Check sheet for the modelled part. Datum: model origin and axes. Units: mm. Face numbers are marked on the shaded views. A direction names the side the tool comes from. Round coordinates to 2 decimals unless told otherwise and drop trailing zeros. Order: outer loops, then holes, each group sorted by start corner. A loop starts at its lowest first (then second) coordinate and runs counter-clockwise, first axis right, second up. Notation, with made-up numbers: (-40, 84.5) -> (19, 84.5) arc R25 cw to (19, 100.5) -> close; hole circle Ø8 at (63, 84.5). An arc over 180 degrees is marked (long way). Answer in a Markdown table with one row per item.
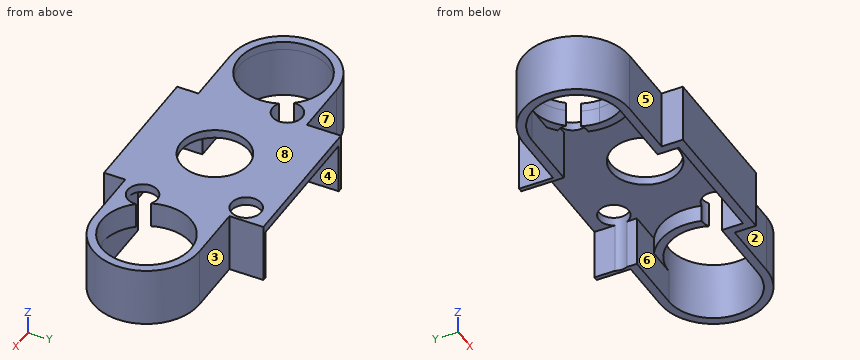
from build123d import *

# Parameters (mm, degrees)
FRONT_PLATE_DEPTH                   = 2
SHELL_DEPTH                         = 12
SHELL_HOLLOW_DEPTH                  = 12
SK_IRRINGS_R                        = 12.5
SK_IRRINGS_R_2                      = 10.5
IR_LED_RINGS_DEPTH                  = 4
LENS_LDR_AND_IR_OPENINGS_DEPTH      = 53.792538299
LENS_LDR_AND_IR_OPENINGS_DEPTH_BACK = 53.792538299
SK_FRONTOPENINGS_R                  = 8
SK_FRONTOPENINGS_R_2                = 3.5
SK_FRONTOPENINGS_R_3                = 10.5
IR_BOARD_NOTCHES_DEPTH              = 53.792538299
IR_BOARD_NOTCHES_DEPTH_BACK         = 53.792538299
SK_IRNOTCHES_R                      = 3.5


with BuildPart() as part:
    # Sk_FrontPlate → Front Plate (new body)
    with BuildSketch(Plane.XY.offset(3)):
        with BuildLine():
            Line((29.79, 18), (16.34, 18))
            Line((16.34, 18), (16.34, 26))
            Line((16.34, 26), (-18.66, 26))
            Line((-18.66, 26), (-18.66, 18))
            Line((-18.66, 18), (-32.11, 18))
            ThreePointArc((-32.11, 18), (-44.61, 5.5), (-32.11, -7))
            Line((-32.11, -7), (-17.66, -7))
            Line((-17.66, -7), (-17.66, -12))
            Line((-17.66, -12), (15.34, -12))
            Line((15.34, -12), (15.34, -7))
            Line((15.34, -7), (29.79, -7))
            ThreePointArc((29.79, -7), (42.29, 5.5), (29.79, 18))
        make_face()
    extrude(amount=-FRONT_PLATE_DEPTH)

    # Sk_ShellOuter → Shell (add)
    with BuildSketch(Plane.XY.offset(1)):
        with BuildLine():
            Line((29.79, 18), (16.34, 18))
            Line((16.34, 18), (16.34, 26))
            Line((16.34, 26), (-18.66, 26))
            Line((-18.66, 26), (-18.66, 18))
            Line((-18.66, 18), (-32.11, 18))
            ThreePointArc((-32.11, 18), (-44.61, 5.5), (-32.11, -7))
            Line((-32.11, -7), (-17.66, -7))
            Line((-17.66, -7), (-17.66, -12))
            Line((-17.66, -12), (15.34, -12))
            Line((15.34, -12), (15.34, -7))
            Line((15.34, -7), (29.79, -7))
            ThreePointArc((29.79, -7), (42.29, 5.5), (29.79, 18))
        make_face()
    extrude(amount=-SHELL_DEPTH)

    # Sk_ShellInner → Shell Hollow (cut)
    with BuildSketch(Plane.XY.offset(1)):
        with BuildLine():
            Line((29.79, 16), (15.34, 16))
            Line((15.34, 16), (15.34, 27))
            Line((15.34, 27), (-17.66, 27))
            Line((-17.66, 27), (-17.66, 16))
            Line((-17.66, 16), (-32.11, 16))
            ThreePointArc((-32.11, 16), (-42.61, 5.5), (-32.11, -5))
            Line((-32.11, -5), (-15.66, -5))
            Line((-15.66, -5), (-15.66, -10))
            Line((-15.66, -10), (13.34, -10))
            Line((13.34, -10), (13.34, -5))
            Line((13.34, -5), (29.79, -5))
            ThreePointArc((29.79, -5), (40.29, 5.5), (29.79, 16))
        make_face()
    extrude(amount=-SHELL_HOLLOW_DEPTH, mode=Mode.SUBTRACT)

    # Sk_IRRings → IR LED Rings (add)
    # profile 1 of 2: a face of its own
    with BuildSketch(Plane.XY.offset(1)):
        with Locations((-32.11, 5.5)):
            Circle(SK_IRRINGS_R)
        with Locations((-32.11, 5.5)):
            Circle(SK_IRRINGS_R_2, mode=Mode.SUBTRACT)
    # profile 2 of 2: a face of its own
    with BuildSketch(Plane.XY.offset(1)):
        with Locations((29.79, 5.5)):
            Circle(SK_IRRINGS_R)
        with Locations((29.79, 5.5)):
            Circle(SK_IRRINGS_R_2, mode=Mode.SUBTRACT)
    extrude(amount=-IR_LED_RINGS_DEPTH)

    # Sk_FrontOpenings → Lens, LDR and IR Openings (cut, two sides: drawn at the far end of the back side and taken through both)
    with BuildSketch(Plane.XY.offset(-LENS_LDR_AND_IR_OPENINGS_DEPTH_BACK)):
        with Locations((-1.11, 5.5)):
            Circle(SK_FRONTOPENINGS_R)
        with Locations((12.15, 19.76)):
            Circle(SK_FRONTOPENINGS_R_2)
        with Locations((-32.11, 5.5)):
            Circle(SK_FRONTOPENINGS_R_3)
        with Locations((29.79, 5.5)):
            Circle(SK_FRONTOPENINGS_R_3)
    extrude(amount=LENS_LDR_AND_IR_OPENINGS_DEPTH + LENS_LDR_AND_IR_OPENINGS_DEPTH_BACK, mode=Mode.SUBTRACT)

    # Sk_IRNotches → IR Board Notches (cut, two sides: drawn at the far end of the back side and taken through both)
    with BuildSketch(Plane.XY.offset(-IR_BOARD_NOTCHES_DEPTH_BACK)):
        with Locations((-20.51, 12.45)):
            Circle(SK_IRNOTCHES_R)
        with Locations((18.19, -1.45)):
            Circle(SK_IRNOTCHES_R)
    extrude(amount=IR_BOARD_NOTCHES_DEPTH + IR_BOARD_NOTCHES_DEPTH_BACK, mode=Mode.SUBTRACT)


solid = part.part
Item 1: Cross-section at C-C (z = -9.75). Record the boundary of the cut face in (x, y).
Result sheet:
| item | result |
|---|---|
| outline | (-32.11, -7) -> (-17.66, -7) -> (-17.66, -12) -> (15.34, -12) -> (15.34, -7) -> (29.79, -7) arc R12.5 ccw to (29.79, 18) -> (16.34, 18) -> (16.34, 26) -> (15.34, 26) -> (15.34, 21.2) arc R3.5 cw to (15.34, 18.32) -> (15.34, 16) -> (29.79, 16) arc R10.5 cw to (29.79, -5) -> (13.34, -5) -> (13.34, -10) -> (-15.66, -10) -> (-15.66, -5) -> (-32.11, -5) arc R10.5 cw to (-32.11, 16) -> (-17.66, 16) -> (-17.66, 26) -> (-18.66, 26) -> (-18.66, 18) -> (-32.11, 18) arc R12.5 ccw to start |
Item 2: Cross-section at D-D (y = 19.76). Record the boundary of the cut face in (x, z), and give its area (3 significant figures).
Result sheet:
| item | result |
|---|---|
| outline | (-18.66, -11) -> (-17.66, -11) -> (-17.66, 1) -> (8.65, 1) -> (8.65, 3) -> (-18.66, 3) -> close; (15.65, -11) -> (16.34, -11) -> (16.34, 3) -> (15.65, 3) -> close |
| area | 76.3 mm^2 |
Item 3: Depth check by flat-ended pin: P1, Ø18.5, axis at x = -1.11, y = 5.5, coming from the -Z side; P2, Ø1.9, axis at y = 17.5, z = -3, coming from the -X side; P3, Ø2.5, axis at y = 24.5, z = -7, coming from the -X side; P4, Ø8, axis at y = 5, z = -5, coming from the -X side. Enter the tip coordinate at first touch or a pass-through.
Result sheet:
| item | result |
|---|---|
| P1 | stops at z = 1 |
| P2 | stops at x = -37.95 |
| P3 | stops at x = -18.66 |
| P4 | stops at x = -44.61 |
Item 4: Mould release check, pull along Y, two halves, no side actions. Record for the marked faces 6, 7 and 8: pulls with the +Y half, pulls with the -Y half, needs draft (parallel to the pull), parting line crosses it, or undercut.
Result sheet:
| item | result |
|---|---|
| face 6 | undercut |
| face 7 | pulls with the +Y half |
| face 8 | needs draft |
Item 5: Cross-section at A-A (x = 12.15). Record the boundary of the cut face in (y, z), and give its area (3 significant figures).
Result sheet:
| item | result |
|---|---|
| outline | (-12, -11) -> (-10, -11) -> (-10, 1) -> (16.26, 1) -> (16.26, 3) -> (-12, 3) -> close; (23.26, 1) -> (26, 1) -> (26, 3) -> (23.26, 3) -> close |
| area | 86.0 mm^2 |
Item 6: Cross-section at B-B (y = 4.5). Record the boundary of the cut face in (x, z).
Result sheet:
| item | result |
|---|---|
| outline | (-44.57, -11) -> (-42.56, -11) -> (-42.56, 3) -> (-44.57, 3) -> close; (-21.66, -3) -> (-19.65, -3) -> (-19.65, 1) -> (-9.05, 1) -> (-9.05, 3) -> (-21.66, 3) -> close; (6.83, 1) -> (17.33, 1) -> (17.33, -3) -> (19.34, -3) -> (19.34, 3) -> (6.83, 3) -> close; (40.24, -11) -> (42.25, -11) -> (42.25, 3) -> (40.24, 3) -> close |
Item 7: Set-up check for the marked faces 1, 2, 3, 4 and 5: record each of +Z, -Z, +X, -X, +Y, -Y from which the full face is reachable in a straight line by a thin tool's end or side.
Result sheet:
| item | result |
|---|---|
| face 1 | +Z, -Z, -X, +Y |
| face 2 | +Z, -Z, +X, -Y |
| face 3 | +Z, -Z, +X, +Y |
| face 4 | -Z, +Y |
| face 5 | +Z, -Z, -X, -Y |
Item 8: Scan lines: line 1 (X direction, y = 5.5, z = 2.05); line 2 (Y direction, x = 29.79, z = -3.75); line 3 (X direction, y = 5.5, z = -5). Record each from-to range of solid material in increasing order. Write a range as [from, to].
Result sheet:
| item | result |
|---|---|
| line 1 | x = [-44.61, -42.61], [-21.61, -9.11], [6.89, 19.29], [40.29, 42.29] |
| line 2 | y = [-7, -5], [16, 18] |
| line 3 | x = [-44.61, -42.61], [40.29, 42.29] |
